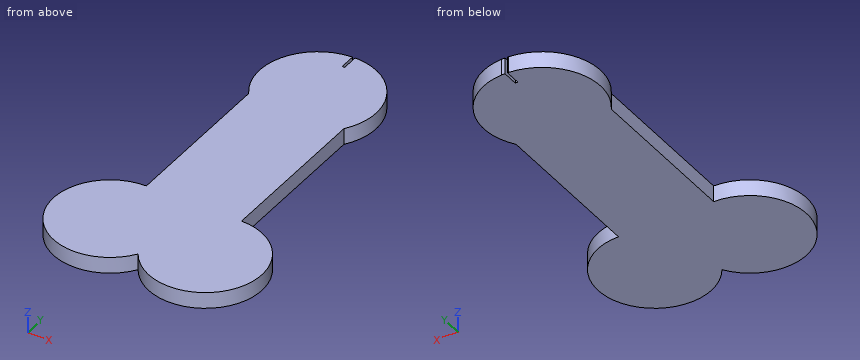
from build123d import *

# Parameters (mm, degrees)
F1_DEPTH = 5


with BuildPart() as f1:
    # F0 (on Top) → F1 (new body)
    with BuildSketch(Plane.XY):
        with BuildLine():
            Line((14.701757, -17.821519), (14.701757, 31.603123))
            ThreePointArc((14.701757, 31.603123), (16.224064, 49.811273), (1.041059, 59.976434))
            Line((1.041059, 59.976434), (0, 59.976434))
            Line((0, 59.976434), (0, 55.009447))
            Line((0, 55.009447), (-0.774187, 55.009447))
            Line((-0.774187, 55.009447), (-0.774187, 59.976434))
            Line((-0.774187, 59.976434), (-1.041059, 59.976434))
            ThreePointArc((-1.041059, 59.976434), (-16.224064, 49.811273), (-14.701757, 31.603123))
            Line((-14.701757, 31.603123), (-14.701757, -17.821519))
            ThreePointArc((-14.701757, -17.821519), (-30.07006, -43.692018), (0, -44.81406))
            ThreePointArc((0, -44.81406), (30.07006, -43.692018), (14.701757, -17.821519))
        make_face()
    extrude(amount=F1_DEPTH)


solid = f1.part
Build history of the part. All positions in model axes, mm. Round coordinates to 2 decimals unless told otherwise and drop trailing zeros. Write each loop counter-clockwise with the first axis right and the second up, starting at its lowest first coordinate (ties: lowest second). Pieces come first, ordered by that corner, then holes. Notation, with made-up numbers: M 58.25,50 L 82.25,50 A20 cw 82.25,64 Z; hole C -5,15.25 d1. An arc over 180 degrees is marked long. Use CSV: the item, a comma, the result in double quotes.
1. Saw through at A-A (z = 4.15). Give the cut face in (x, y), plus the area to 3 significant figures.
Reply:
outline,"M -14.7,-17.82 A17.5 ccw long 0,-44.81 A17.5 ccw long 14.7,-17.82 L 14.7,31.6 A18.01 ccw 1.04,59.98 L 0,59.98 L 0,55.01 L -0.77,55.01 L -0.77,59.98 L -1.04,59.98 A18.01 ccw -14.7,31.6 Z"
area,"4,230 mm²"
2. Saw through at C-C (x = -25). Give the cut face in (y, z).
Reply:
outline,"M -49.47,0 L -21.17,0 L -21.17,5 L -49.47,5 Z"
3. Saw through at B-B (y = -6). Give the cut face in (x, z), plus the area to 3 significant figures.
Reply:
outline,"M -14.7,0 L 14.7,0 L 14.7,5 L -14.7,5 Z"
area,"147 mm²"
4. Wall check: probe 1 along X at (y, z) = (-7, 2.45); probe 2 along X at (y, z) = (-35.5, 2.35); probe 3 along Y at (x, z) = (-15, 4.35). Give the ranges that are in metal, low to high. Write a range as from..to.
Reply:
probe 1,"x = -14.7..14.7"
probe 2,"x = -32.2..32.2"
probe 3,"y = -52.82..-17.82, 32.04..51.96"
5. Flat gauge pins, fed straight in: pin 1 (3 mm diameter, centred on y = 40.5, z = 4, fed in from -X); pin 2 (3 mm diameter, centred on y = 25, z = 3.5, fed in from -X); pin 3 (2.5 mm diameter, centred on y = 56.5, z = 3, fed in from -X). Where does each tip first touch, or does it go through?
Reply:
pin 1,"stops at x = -18.01"
pin 2,"stops at x = -14.7"
pin 3,"stops at x = -12.19"
